from build123d import *

# Parameters (mm, degrees)
F1_DEPTH = 7.62
F3_DEPTH = 25.4


with BuildPart() as f1:
    # F0 (on Top) → F1 (new body)
    with BuildSketch(Plane.XY):
        Polygon((-43.18, -50.8), (50.8, -50.8), (50.8, -43.18), (-41.383949, -43.18), (-43.18, -43.18), align=None)
        Polygon((-49.003949, -50.8), (-43.18, -50.8), (-43.18, -43.18), (-50.8, -43.18), (-50.8, -49.003949), (-50.8, -50.8), align=None)
        Polygon((-41.383949, -43.18), (50.8, -43.18), (50.8, 42.910773), (50.8, 49.003949), (44.706825, 42.910773), align=None)
        Polygon((-50.8, -43.18), (-43.18, -43.18), (-43.18, -41.383949), (-43.18, 50.8), (-50.8, 50.8), align=None)
        Polygon((-43.18, 50.8), (-43.18, -41.383949), (42.9001, 44.696152), (49.003949, 50.8), (42.9001, 50.8), align=None)
        Polygon((44.706825, 42.910773), (50.8, 49.003949), (50.8, 50.8), (49.003949, 50.8), (42.9001, 44.696152), (44.685479, 42.910773), align=None)
    extrude(amount=F1_DEPTH)

    # F2 (on face) → F3 (join)
    with BuildSketch(Plane.XY.offset(7.62)):
        Polygon((-50.8, -43.18), (-50.8, -50.8), (-43.18, -50.8), (50.8, -50.8), (50.8, -43.18), (-41.383949, -43.18), (-43.18, -43.18), (-43.18, -41.383949), (-43.18, 50.8), (-50.8, 50.8), align=None)
    extrude(amount=F3_DEPTH)


solid = f1.part
Read the model definition and answer for the solid it produces. Units are mm, in the model's axes. Give positions to 0.01 mm unless a question says otherwise; leave off trailing zeros. Write each loop counter-clockwise with the first axis right and the second up, starting at its lowest first coordinate (ties: lowest second). Pieces come first, ordered by that corner, then holes. Notation, with made-up numbers: (32.25, -17) -> (40.25, -17) arc R24 cw to (40.25, 14) -> close; hole circle Ø4 at (2.5, 81.5). An arc over 180 degrees is marked (long way). Answer as a JSON object with one key per item and string values. Group by question number.
1) The mould has two halves that part along X. Classify faces 1 (the flat face through (-0.743, 1.054, 3.757)), 2 (the flat face through (50.8, -12, 7)), 3 (the flat face through (3, 15, 7.62)), 4 (the flat face through (2.264, 0.468, 3.757)): +X half, -X half, draft (parallel to the pull), parting line (faces both ways), or undercut.
2) Find section B-B (x = 2). Write down the section's boundary in (y, z).
3) Find section C-C (y = -37). Write down the section's boundary in (x, z).
4) Each of these flat-tipped pins is pushed along its axis until it touches: P1, Ø5, axis at x = -8, y = -21, coming from the +Z side; P2, Ø2, axis at y = 37, z = 25.5, coming from the +X side; P3, Ø1.5, axis at x = 34, z = 29.5, coming from the +Y side. Where does it stop, or does it pass through?
5) Find section D-D (z = 30). Write down the section's boundary in (x, y).
6) Consider L1, parallel to X at y = 47, z = 23.5; L2, parallel to Z at x = -23, y = 42.5. Determine where each line is inside the solid, lowest interval first. Write a range as from..to.
Values follow:
{
 "1": {"face 1": "undercut", "face 2": "+X half", "face 3": "draft", "face 4": "undercut"},
 "2": {"outline": "(-50.8, 0) -> (0.2, 0) -> (0.2, 7.62) -> (-43.18, 7.62) -> (-43.18, 33.02) -> (-50.8, 33.02) -> close; (3.8, 0) -> (50.8, 0) -> (50.8, 7.62) -> (3.8, 7.62) -> close"},
 "3": {"outline": "(-50.8, 0) -> (-38.8, 0) -> (-38.8, 7.62) -> (-43.18, 7.62) -> (-43.18, 33.02) -> (-50.8, 33.02) -> close; (-35.2, 0) -> (50.8, 0) -> (50.8, 7.62) -> (-35.2, 7.62) -> close"},
 "4": {"P1": "stops at z = 7.62", "P2": "stops at x = -43.18", "P3": "stops at y = -43.18"},
 "5": {"outline": "(-50.8, -50.8) -> (50.8, -50.8) -> (50.8, -43.18) -> (-43.18, -43.18) -> (-43.18, 50.8) -> (-50.8, 50.8) -> close"},
 "6": {"L1": "x = -50.8..-43.18", "L2": "z = 0..7.62"}
}
